Input: dimensioned drawing with shaded views. Units: mm. Origin: part minimum x, y, z. A direction names the side the tool comes from. Give positions to 0.01 mm unless a question says otherwise; leave off trailing zeros. Write each loop counter-clockwise with the first axis right and the second up, starting at its lowest first coordinate (ties: lowest second). Pieces come first, ordered by that corner, then holes. Notation, with made-up numbers: (10, -5.5) - (60, -5.5) arc R25 cw to (60, 28.5) - close; hole circle Ø8 at (24, 35.5). An arc over 180 degrees is marked (long way). Answer as a JSON object with one key per item and string values. Group by question number.
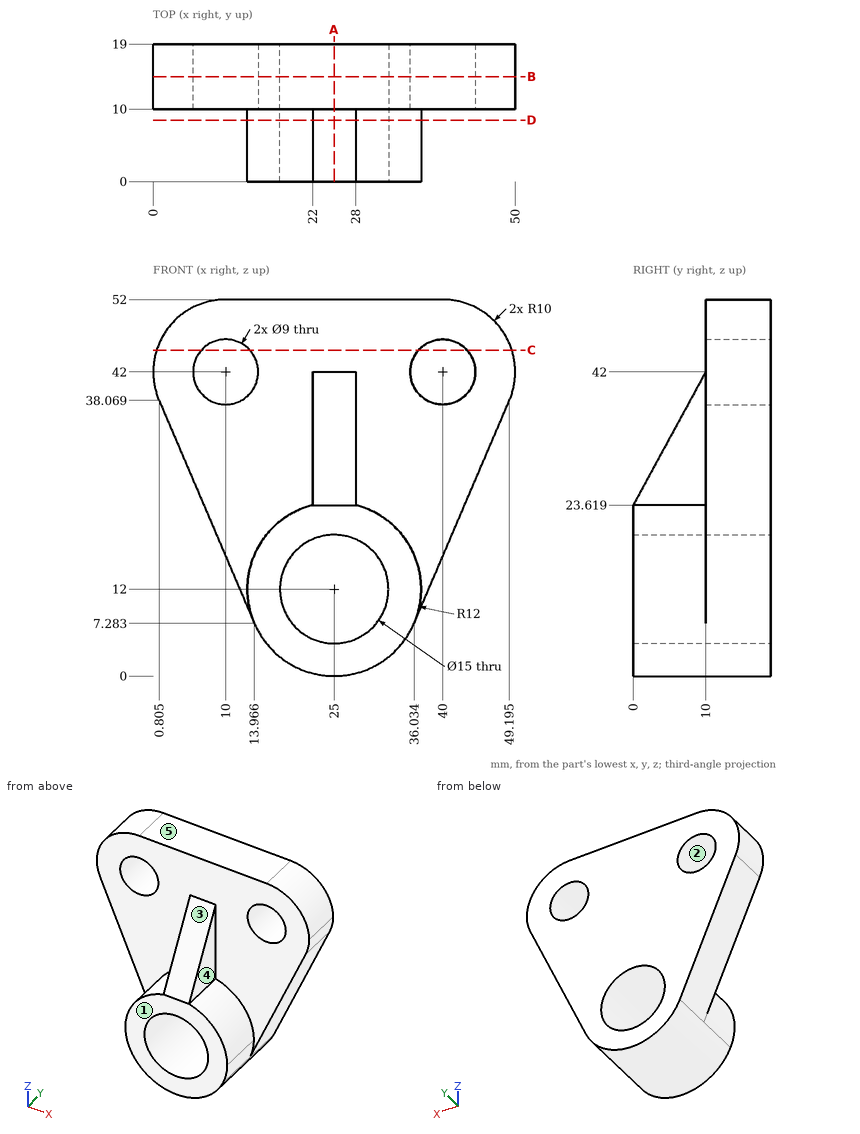
Q1. Ray query, probe 1 along Y at (x, z) = (42.5, 29.5); probe 2 along Z at (x, y) = (37.5, 16.75); probe 3 along X at (y, z) = (17.25, 18) (1 decimal). Return the intervals inside material, ascending. Write a range as [from, to].
Q2. Reachability of the marked faces 4 and 5 from +Z, -Z, +X, -X, +Y, -Y: full face, straight path, thin tool, end or side. Return the list, or none.
Q3. First-contact query: pin 1 Ø5 at (y, z) = (14, 36.5) entering from +X; pin 2 Ø3 at (y, z) = (5, 32) entering from -X; pin 3 Ø5 at (x, y) = (29, 10) entering from -Z. Flat tips, straight axial feed; report the tip coordinate or a pass-through.
Q4. Section B-B on y = 14.5. Return the cut outline in (x, z) (3 decimals).
Q5. Section D-D on y = 8.5. Return the cut outline in (x, z), then the cut area to 3 significant figures.
Q6. Draft query along Z for the marked faces 1, 2 and 3. Return one class per face: released by +Z, released by -Z, zero draft, split by the parting line, or undercut.
Q7. Section A-A on x = 25. Return the cut outline in (y, z), then the cut area to 3 significant figures.
Q8. Section C-C on z = 45. Return the cut outline in (x, y), then the cut area to 3 significant figures.
Taken from the geometry:
{
 "1": {"probe 1": "y = [10, 19]", "probe 2": "z = [10.71, 38.26], [45.74, 52]", "probe 3": "x = [9.4, 20.5], [29.5, 40.6]"},
 "2": {"face 4": "+Z, +X, -Y", "face 5": "+Z, +X, -X, +Y, -Y"},
 "3": {"pin 1": "stops at x = 49.54", "pin 2": "stops at x = 22", "pin 3": "stops at z = 0.09"},
 "4": {"outline": "(0.805, 38.069) - (13.966, 7.283) arc R12 ccw to (36.034, 7.283) - (49.195, 38.069) arc R10 ccw to (50, 42) arc R10 ccw to (40, 52) - (10, 52) arc R10 ccw to start; hole circle Ø9 at (10, 42); hole circle Ø15 at (25, 12); hole circle Ø9 at (40, 42)"},
 "5": {"outline": "(22, 23.62) arc R12 ccw (long way) to (36.03, 7.28) arc R12 ccw to (37, 12) arc R12 ccw to (28, 23.62) - (28, 39.24) - (22, 39.24) - close; hole circle Ø15 at (25, 12)", "area": "368 mm²"},
 "6": {"face 1": "zero draft", "face 2": "undercut", "face 3": "released by +Z"},
 "7": {"outline": "(0, 0) - (19, 0) - (19, 4.5) - (0, 4.5) - close; (0, 19.5) - (19, 19.5) - (19, 52) - (10, 52) - (10, 42) - (0, 23.62) - close", "area": "511 mm²"},
 "8": {"outline": "(0.46, 10) - (6.65, 10) - (6.65, 19) - (0.46, 19) - close; (13.35, 10) - (36.65, 10) - (36.65, 19) - (13.35, 19) - close; (43.35, 10) - (49.54, 10) - (49.54, 19) - (43.35, 19) - close", "area": "321 mm²"}
}
